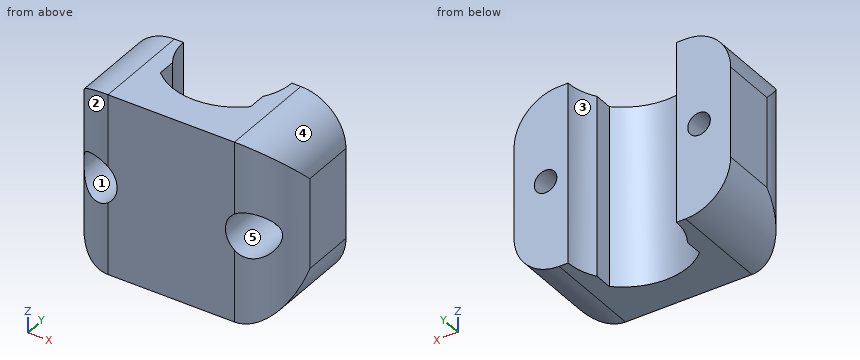
```python
from build123d import *

# Parameters (mm, degrees)
BOSS_EXTRUDE1_DEPTH     = 10
SKETCH2_W               = 10
SKETCH2_H               = 5.318834459
CUT_EXTRUDE1_DEPTH      = 11
CUT_EXTRUDE1_DEPTH_BACK = 11
SKETCH3_R               = 1.25
CUT_EXTRUDE2_DEPTH      = 17
FILLET1_R               = 5
CUT_EXTRUDE3_DEPTH      = 11
CUT_EXTRUDE3_DEPTH_BACK = 11
SKETCH5_R               = 2.5
CUT_EXTRUDE4_DEPTH      = 6


with BuildPart() as part:
    # Sketch1 → Boss-Extrude1 (new body, symmetric)
    with BuildSketch(Plane.XY):
        with BuildLine():
            Line((12, 0), (6, 0))
            ThreePointArc((6, 0), (0, -6), (-6, 0))
            Line((-6, 0), (-12, 0))
            Line((-12, 0), (-12, -11))
            Line((-12, -11), (12, -11))
            Line((12, -11), (12, 0))
        make_face()
    extrude(amount=BOSS_EXTRUDE1_DEPTH, both=True)

    # Sketch2 → Cut-Extrude1 (cut, two sides)
    with BuildSketch(Plane.XY) as cut_extrude1_sk:
        with BuildLine():
            Line((5, -5.318834459), (-5, -5.318834459))
            ThreePointArc((-5, -5.318834459), (0, -7.3), (5, -5.318834459))
        make_face()
        with Locations((0, -2.65941723)):
            Rectangle(SKETCH2_W, SKETCH2_H)
    extrude(amount=CUT_EXTRUDE1_DEPTH, mode=Mode.SUBTRACT)
    extrude(cut_extrude1_sk.sketch, amount=-CUT_EXTRUDE1_DEPTH_BACK, mode=Mode.SUBTRACT)

    # Sketch3 → Cut-Extrude2 (cut)
    with BuildSketch(Plane(origin=(0, 0, 0), x_dir=(1, 0, 0), z_dir=(0, 1, 0))):
        with Locations((-8.5, 0)):
            Circle(SKETCH3_R)
        with Locations((8.5, 0)):
            Circle(SKETCH3_R)
    extrude(amount=-CUT_EXTRUDE2_DEPTH, mode=Mode.SUBTRACT)

    # Fillet1
    fillet1_edges = [part.edges().sort_by_distance(p)[0] for p in [
        (12, -5.5, 10),
        (-12, -5.5, 10),
        (-12, -5.5, -10),
        (12, -5.5, -10),
    ]]
    fillet(fillet1_edges, radius=FILLET1_R)

    # Sketch4 → Cut-Extrude3 (cut, two sides)
    with BuildSketch(Plane.XY) as cut_extrude3_sk:
        with BuildLine():
            ThreePointArc((7, -11), (10.535533906, -9.535533906), (12, -6))
            Line((12, -6), (12, -11))
            Line((12, -11), (7, -11))
        make_face()
        with BuildLine():
            ThreePointArc((-12, -6), (-10.535533906, -9.535533906), (-7, -11))
            Line((-7, -11), (-12, -11))
            Line((-12, -11), (-12, -6))
        make_face()
    extrude(amount=CUT_EXTRUDE3_DEPTH, mode=Mode.SUBTRACT)
    extrude(cut_extrude3_sk.sketch, amount=-CUT_EXTRUDE3_DEPTH_BACK, mode=Mode.SUBTRACT)

    # Sketch5 → Cut-Extrude4 (cut)
    with BuildSketch(Plane.XZ.offset(11)):
        with Locations((-8.5, 0)):
            Circle(SKETCH5_R)
        with Locations((8.5, 0)):
            Circle(SKETCH5_R)
    extrude(amount=-CUT_EXTRUDE4_DEPTH, mode=Mode.SUBTRACT)


solid = part.part
```
Verification items for the finished model (mm, model axes). Face numbers are marked on the shaded views. A direction names the side the tool comes from. Round coordinates to 2 decimals unless told otherwise and drop trailing zeros. Order: outer loops, then holes, each group sorted by start corner. A loop starts at its lowest first (then second) coordinate and runs counter-clockwise, first axis right, second up.
1) Cross-section at B-B, the plane z = 0. Record the cut outline in (x, y).
Geometry says:
outline: (-12, -6) arc R5 ccw to (-11, -9) - (-11, -5) - (-9.75, -5) - (-9.75, 0) - (-12, 0) - close; (-7.25, -5) - (-6, -5) - (-6, -11) - (6, -11) - (6, -5) - (7.25, -5) - (7.25, 0) - (6, 0) arc R6 cw to (5, -3.32) - (5, -5.32) arc R7.3 cw to (-5, -5.32) - (-5, -3.32) arc R6 cw to (-6, 0) - (-7.25, 0) - close; (9.75, -5) - (11, -5) - (11, -9) arc R5 ccw to (12, -6) - (12, 0) - (9.75, 0) - close
2) Cross-section at C-C, the plane x = -8.25. Record the cut outline in (y, z).
Geometry says:
outline: (-10.84, -9.84) - (0, -9.84) - (0, -1.22) - (-5, -1.22) - (-5, -2.49) - (-10.84, -2.49) - close; (-10.84, 2.49) - (-5, 2.49) - (-5, 1.22) - (0, 1.22) - (0, 9.84) - (-10.84, 9.84) - close
3) Depth check by flat-ended pin: pin 1 (10 mm diameter, centred on x = 8.5, z = 5, fed in from +Y); pin 2 (1 mm diameter, centred on x = -3, z = 2.5, fed in from +Y); pin 3 (1.5 mm diameter, centred on x = -9.5, z = 0, fed in from -Y); pin 4 (4 mm diameter, centred on x = 9.5, z = 0, fed in from -Y). Enter the tip coordinate at first touch or a pass-through.
Geometry says:
pin 1: stops at y = 0
pin 2: stops at y = -6.41
pin 3: stops at y = -5
pin 4: stops at y = -9.9
4) Cross-section at A-A, the plane y = -7. Record the cut outline in (x, z), plus the area to 3 significant figures.
Geometry says:
outline: (-11.9, -6) arc R5 ccw to (-7, -10) - (-2.07, -10) - (-2.07, 10) - (-7, 10) arc R5 ccw to (-11.9, 6) - close; (2.07, -10) - (7, -10) arc R5 ccw to (11.9, -6) - (11.9, 6) arc R5 ccw to (7, 10) - (2.07, 10) - close; hole circle Ø5 at (-8.5, 0); hole circle Ø5 at (8.5, 0)
area: 334 mm2
5) Draft check along Z on the marked faces 3, 4 and 5. Enter one of: +Z half, -Z half, draft (parallel to the pull), parting line (faces both ways), or undercut.
Geometry says:
face 3: draft
face 4: +Z half
face 5: undercut
6) Cross-section at D-D, the plane z = 3.5. Record the cut outline in (x, y).
Geometry says:
outline: (-12, -6) arc R5 ccw to (-7, -11) - (7, -11) arc R5 ccw to (12, -6) - (12, 0) - (6, 0) arc R6 cw to (5, -3.32) - (5, -5.32) arc R7.3 cw to (-5, -5.32) - (-5, -3.32) arc R6 cw to (-6, 0) - (-12, 0) - close
7) Material ranges on line 1 (X direction, y = -5, z = -4.25); line 2 (X direction, y = -9, z = -1.5); line 3 (X direction, y = -1.15, z = 0), recorded low to high.
Geometry says:
line 1: x = -12 to -5, 5 to 12
line 2: x = -11 to -10.5, -6.5 to 6.5, 10.5 to 11
line 3: x = -12 to -9.75, -7.25 to -5.89, 5.89 to 7.25, 9.75 to 12
8) Tool access check on the marked faces 1 and 2. Record the directions out of +Z, -Z, +X, -X, +Y, -Y that give a thin tool (end or side, any length) a straight path to the whole face; none if there is none.
Geometry says:
face 1: -Y
face 2: +Z, -Z, -X, -Y
